Verification items for the finished model (mm, model axes). A direction names the side the tool comes from. Coordinates: 2 decimals unless noted, no trailing zeros. Order: outer loops, then holes, each group sorted by start corner. A loop starts at its lowest first (then second) coordinate and runs counter-clockwise, first axis right, second up. Notation, with made-up numbers: M 63,86 L 82,86 A11 ccw 82,90 Z; hole C 78,55 d3. An arc over 180 degrees is marked long. Return JSON: item names as keys, results as strings.
```python
from build123d import *

# Parameters (mm, degrees)
F1_W     = 20
F1_H     = 14.6167501807
F1_H_2   = 5
F2_DEPTH = 5


with BuildPart() as f2:
    # F1 (on Right) → F2 (new body)
    with BuildSketch(Plane.YZ):
        Polygon((0, 60), (0, 0), (10, 0), (30, 0), (55, 0), (75, 0), (83.4, 0), (83.4, 2.5), (82.25, 2.5), (82.25, 5), (85, 5), (87.75, 5), (87.75, 2.5), (86.6, 2.5), (86.6, 0), (95, 0), (115, 0), (140, 0), (160, 0), (170, 0), (170, 60), (160, 60), (140, 60), (115, 60), (95, 60), (86.6, 60), (86.6, 57.5), (87.75, 57.5), (87.75, 55), (85, 55), (82.25, 55), (82.25, 57.5), (83.4, 57.5), (83.4, 60), (75, 60), (55, 60), (30, 60), (10, 60), align=None)
        with Locations((20, -7.3083750904)):
            Rectangle(F1_W, F1_H)
        with Locations((20, 62.5)):
            Rectangle(F1_W, F1_H_2)
        with Locations((65, -2.5)):
            Rectangle(F1_W, F1_H_2)
        with Locations((65, 62.5)):
            Rectangle(F1_W, F1_H_2)
        with Locations((105, -2.5)):
            Rectangle(F1_W, F1_H_2)
        with Locations((105, 62.5)):
            Rectangle(F1_W, F1_H_2)
        with Locations((150, -7.3083750904)):
            Rectangle(F1_W, F1_H)
        with Locations((150, 62.5)):
            Rectangle(F1_W, F1_H_2)
    extrude(amount=F2_DEPTH)


solid = f2.part
```
Q1. Cross-section at B-B, the plane y = 51. Record the boundary of the cut face in (x, z), and give its area (3 significant figures).
Values:
{"outline": "M 0,0 L 5,0 L 5,60 L 0,60 Z", "area": "300 mm^2"}
Q2. Cross-section at A-A, the plane y = 70. Record the boundary of the cut face in (x, z).
Values:
{"outline": "M 0,-5 L 5,-5 L 5,65 L 0,65 Z"}
Q3. Draft check along Y on faces 1 (the face through (2, 75, -3)), 2 (the face through (2, 10, -7)), 3 (the face through (2, 165, 60)). Enter one of: pulls with the +Y half, pulls with the -Y half, needs draft (parallel to the pull), parting line crosses it, or undercut.
Values:
{"face 1": "undercut", "face 2": "pulls with the -Y half", "face 3": "needs draft"}
Q4. Material ranges on line 1 along Y through (x, z) = (4.2, -1); line 2 along Z through (x, y) = (3.7, 68.5); line 3 along Y through (x, z) = (1.2, 1), recorded low to high.
Values:
{"line 1": "10 to 30, 55 to 75, 95 to 115, 140 to 160", "line 2": "-5 to 65", "line 3": "0 to 83.4, 86.6 to 170"}
Q5. Go/stop test with flat-tipped pins: pin 1 (4 mm diameter, centred on y = 23, z = 10, fed in from -X); pin 2 (1.5 mm diameter, centred on x = 3.5, z = 63, fed in from -Y); pin 3 (1.5 mm diameter, centred on x = 3, y = 121.5, fed in from -Z); pin 4 (2.5 mm diameter, centred on x = 2.5, z = -3.5, fed in from +Y). Record where each tip stops, or that it passes through.
Values:
{"pin 1": "x = 0", "pin 2": "y = 10", "pin 3": "z = 0", "pin 4": "y = 160"}
Q6. Tool access check on faces 4 (the face through (2, 30, -7)), 5 (the face through (2, 85, 5)), 6 (the face through (2, 160, 62)), 7 (the face through (2, 30, 62)). Record the directions out of +Z, -Z, +X, -X, +Y, -Y that give a thin tool (end or side, any length) a straight path to the whole face; none if there is none.
Values:
{"face 4": "-Z, +X, -X", "face 5": "+X, -X", "face 6": "+Z, +X, -X, +Y", "face 7": "+Z, +X, -X"}
